```python
from build123d import *

# Parameters (mm, degrees)
SKETCH1_W           = 63.5
SKETCH1_H           = 19.05
SKETCH1_R           = 3.9878
BOSS_EXTRUDE1_DEPTH = 25.4
SKETCH2_R           = 2
CUT_EXTRUDE1_DEPTH  = 6.35
SKETCH3_W           = 25.4
SKETCH3_H           = 19.05
CUT_EXTRUDE2_DEPTH  = 22.225
SKETCH6_R           = 0.95
SKETCH6_R_2         = 3.5
CUT_EXTRUDE3_DEPTH  = 4.175


with BuildPart() as part:
    # Sketch1 → Boss-Extrude1 (new body)
    with BuildSketch(Plane.XY):
        Rectangle(SKETCH1_W, SKETCH1_H)
        with Locations((-22.225, -3.175)):
            Circle(SKETCH1_R, mode=Mode.SUBTRACT)
        with Locations((22.225, -3.175)):
            Circle(SKETCH1_R, mode=Mode.SUBTRACT)
    extrude(amount=-BOSS_EXTRUDE1_DEPTH)

    # Sketch2 → Cut-Extrude1 (cut)
    with BuildSketch(Plane.ZY.offset(31.75)):
        with Locations((-12.7, 3.175)):
            Circle(SKETCH2_R)
    cut_extrude1 = extrude(amount=-CUT_EXTRUDE1_DEPTH, mode=Mode.SUBTRACT)

    # Mirror1: Cut-Extrude1 across plane
    add(cut_extrude1.mirror(Plane.ZY), mode=Mode.SUBTRACT)

    # Sketch3 → Cut-Extrude2 (cut)
    with BuildSketch(Plane.XY):
        Rectangle(SKETCH3_W, SKETCH3_H)
    extrude(amount=-CUT_EXTRUDE2_DEPTH, mode=Mode.SUBTRACT)

    # Sketch6 → Cut-Extrude3 (cut, through all)
    with BuildSketch(Plane.XY.offset(-22.225)):
        with Locations((-7.5, 0)):
            Circle(SKETCH6_R)
        with Locations((7.5, 0)):
            Circle(SKETCH6_R)
        Circle(SKETCH6_R_2)
    extrude(amount=-CUT_EXTRUDE3_DEPTH, mode=Mode.SUBTRACT)


solid = part.part
```
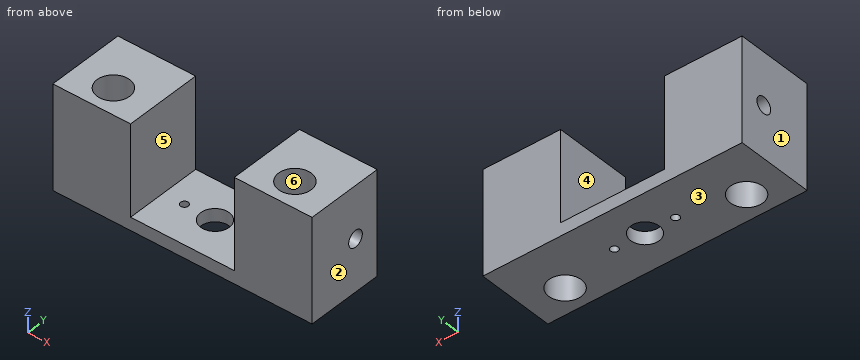
Check sheet for the modelled part. Datum: model origin and axes. Units: mm. Face numbers are marked on the shaded views. A direction names the side the tool comes from. Round coordinates to 2 decimals unless told otherwise and drop trailing zeros. Order: outer loops, then holes, each group sorted by start corner. A loop starts at its lowest first (then second) coordinate and runs counter-clockwise, first axis right, second up.
1) Section check C-C (y = 2.5). Record the boundary of the cut face in (x, z) (3 decimals).
2) Mould release check, pull along X, two halves, no side actions. Record for the marked faces 1, 2, 3 and 4: +X half, -X half, draft (parallel to the pull), parting line (faces both ways), or undercut.
3) Scan lines: line 1 (X direction, y = -3, z = -12.25); line 2 (Y direction, x = -30, z = -12.7) (3 decimals); line 3 (X direction, y = -2.5, z = -7.25). Record each from-to range of solid material in increasing order.
4) Section check B-B (z = -20.25). Record the boundary of the cut face in (x, y) (3 decimals), and give its area (3 significant figures).
5) Go/stop test with flat-tipped pins: pin 1 Ø10 at (x, z) = (6, -3) entering from +Y; pin 2 Ø3 at (x, y) = (7.5, 0) entering from +Z (3 decimals); pin 3 Ø2 at (y, z) = (3, -12.5) entering from -X; pin 4 Ø3 at (y, z) = (3.175, -12.7) entering from +X. Record where each tip stops, or that it passes through.
6) Section check A-A (x = 7.5). Record the boundary of the cut face in (y, z) (3 decimals), and give its area (3 significant figures).
7) Section check D-D (x = 0). Record the boundary of the cut face in (y, z) (3 decimals).
8) Tool access check on the marked faces 5 and 6. Record the directions out of +Z, -Z, +X, -X, +Y, -Y that give a thin tool (end or side, any length) a straight path to the whole face; none if there is none.
Result:
1. outline: (-31.75, -25.4) - (-2.449, -25.4) - (-2.449, -22.225) - (-12.7, -22.225) - (-12.7, 0) - (-31.75, 0) - (-31.75, -10.817) - (-25.4, -10.817) - (-25.4, -14.583) - (-31.75, -14.583) - close; (2.449, -25.4) - (31.75, -25.4) - (31.75, -14.583) - (25.4, -14.583) - (25.4, -10.817) - (31.75, -10.817) - (31.75, 0) - (12.7, 0) - (12.7, -22.225) - (2.449, -22.225) - close
2. face 1: -X half
2. face 2: +X half
2. face 3: draft
2. face 4: undercut
3. line 1: x = -31.75 to -26.21, -18.24 to -12.7, 12.7 to 18.24, 26.21 to 31.75
3. line 2: y = -9.525 to 1.175, 5.175 to 9.525
3. line 3: x = -31.75 to -26.16, -18.29 to -12.7, 12.7 to 18.29, 26.16 to 31.75
4. outline: (-31.75, -9.525) - (-12.7, -9.525) - (-12.7, 9.525) - (-31.75, 9.525) - close; (12.7, -9.525) - (31.75, -9.525) - (31.75, 9.525) - (12.7, 9.525) - close; hole circle Ø7.976 at (-22.225, -3.175); hole circle Ø7.976 at (22.225, -3.175)
4. area: 626 mm2
5. pin 1: passes through
5. pin 2: stops at z = -22.225
5. pin 3: stops at x = -25.4
5. pin 4: stops at x = 25.4
6. outline: (-9.525, -25.4) - (-0.95, -25.4) - (-0.95, -22.225) - (-9.525, -22.225) - close; (0.95, -25.4) - (9.525, -25.4) - (9.525, -22.225) - (0.95, -22.225) - close
6. area: 54.5 mm2
7. outline: (-9.525, -25.4) - (-3.5, -25.4) - (-3.5, -22.225) - (-9.525, -22.225) - close; (3.5, -25.4) - (9.525, -25.4) - (9.525, -22.225) - (3.5, -22.225) - close
8. face 5: +Z, +Y, -Y
8. face 6: +Z, -Z
